Check sheet for the modelled part. Datum: model origin and axes. Units: mm. Face numbers are marked on the shaded views. Give positions to 0.01 mm unless a question says otherwise; leave off trailing zeros. Order: outer loops, then holes, each group sorted by start corner. A loop starts at its lowest first (then second) coordinate and runs counter-clockwise, first axis right, second up.
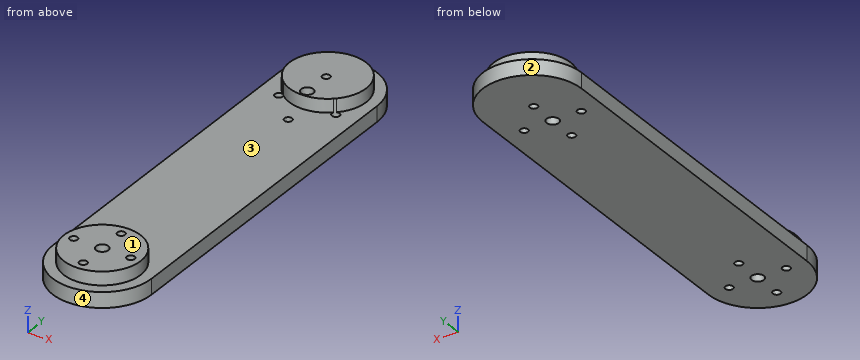
```python
from build123d import *

# Parameters (mm, degrees)
SKETCH_1_R               = 24.9
EXTRUDE_1_DEPTH          = 8.7
EXTRUDE_2_DEPTH          = 10
SKETCH_5_R               = 24.9
EXTRUDE_4_DEPTH          = 8.7
CUT_EXTRUDE_1_DEPTH      = 255.710993088
CUT_EXTRUDE_1_DEPTH_BACK = 255.710993088
SKETCH_2_R               = 4
SKETCH_2_R_2             = 2.5


with BuildPart() as part:
    # 草图1 → 凸台-拉伸1 (new body)
    with BuildSketch(Plane.XY):
        Circle(SKETCH_1_R)
    extrude(amount=EXTRUDE_1_DEPTH)

    # 草图3 → 凸台-拉伸2 (add)
    with BuildSketch(Plane(origin=(0, 0, 0), x_dir=(-1, 0, 0), z_dir=(0, 0, -1))):
        with BuildLine():
            Line((-32, 0), (-32, 220))
            ThreePointArc((-32, 220), (0, 252), (32, 220))
            Line((32, 220), (32, 0))
            ThreePointArc((32, 0), (0, -32), (-32, 0))
        make_face()
    extrude(amount=EXTRUDE_2_DEPTH)

    # 草图5 → 凸台-拉伸4 (add)
    with BuildSketch(Plane.XY):
        with Locations(Location((0, 220, 0), (0, 0, 180))):
            Circle(SKETCH_5_R)
    extrude(amount=EXTRUDE_4_DEPTH)

    # 草图2 → 切除-拉伸1 (cut, two sides: drawn at the far end of the back side and taken through both)
    with BuildSketch(Plane.XY.offset(8.7).offset(-CUT_EXTRUDE_1_DEPTH_BACK)):
        Circle(SKETCH_2_R)
        with Locations((0, 18.5)):
            Circle(SKETCH_2_R_2)
        with Locations((-18.5, 0)):
            Circle(SKETCH_2_R_2)
        with Locations((18.5, 0)):
            Circle(SKETCH_2_R_2)
        with Locations((0, -18.5)):
            Circle(SKETCH_2_R_2)
        with Locations((0, 218.5)):
            Circle(SKETCH_2_R_2)
        with Locations((0, 200)):
            Circle(SKETCH_2_R)
        with Locations((0, 181.5)):
            Circle(SKETCH_2_R_2)
        with Locations((-18.5, 200)):
            Circle(SKETCH_2_R_2)
        with Locations((18.5, 200)):
            Circle(SKETCH_2_R_2)
    extrude(amount=CUT_EXTRUDE_1_DEPTH + CUT_EXTRUDE_1_DEPTH_BACK, mode=Mode.SUBTRACT)


solid = part.part
```
(1) Sectioned sample at A-A (z = 4.75). Count the separate pieces of the cut face and the enclosed holes in it, plus the area to 3 significant figures.
(2) Go/stop test with flat-tipped pins: P1, Ø6, axis at x = 18.5, y = 200, coming from the +Z side; P2, Ø10, axis at x = -19.5, y = 128.5, coming from the +Z side; P3, Ø8, axis at x = 21.5, z = 2.5, coming from the +Y side; P4, Ø1, axis at x = -9, z = 1.5, coming from the +Y side. Record where each tip stops, or that it passes through.
(3) Thickness scan on L1, parallel to X at y = 218.5, z = -1.25; L2, parallel to X at y = 200, z = -0.5; L3, parallel to Y at x = 18.5, z = 4. Record the ranges inside material, lowest first.
(4) Sectioned sample at B-B (y = -18.5). Enter the section's corners in (x, z).
(5) Release check for a two-part mould opening along Y. For the marked faces 1, 2, 3 and 4 record: released by +Y, released by -Y, zero draft, split by the parting line, or undercut.
(6) Sectioned sample at D-D (y = 143). Enter the section's corners in (x, z), plus the area to 3 significant figures.
Values follow:
1. separate pieces: 2
1. enclosed holes: 7
1. area: 3,700 mm2
2. P1: stops at z = 8.7
2. P2: stops at z = 0
2. P3: stops at y = 246.2
2. P4: stops at y = 243.4
3. L1: x = -32 to -2.5, 2.5 to 32
3. L2: x = -32 to -21, -16 to -4, 4 to 16, 21 to 32
3. L3: y = -16.67 to -2.5, 2.5 to 16.67, 203.33 to 236.67
4. outline: (-26.11, -10) - (-2.5, -10) - (-2.5, 8.7) - (-16.67, 8.7) - (-16.67, 0) - (-26.11, 0) - close; (2.5, -10) - (26.11, -10) - (26.11, 0) - (16.67, 0) - (16.67, 8.7) - (2.5, 8.7) - close
5. face 1: zero draft
5. face 2: released by +Y
5. face 3: undercut
5. face 4: released by -Y
6. outline: (-32, -10) - (32, -10) - (32, 0) - (-32, 0) - close
6. area: 640 mm2
